Source: CAD feature listing. Evaluate the final solid. Frame: model axes, mm. Coordinates: 2 decimals unless noted, no trailing zeros. Order: outer loops, then holes, each group sorted by start corner. A loop starts at its lowest first (then second) coordinate and runs counter-clockwise, first axis right, second up. Notation, with made-up numbers: (64, -37) -> (78, -37) arc R12 ccw to (78, -23) -> close; hole circle Ø5 at (-24.5, 24.25). An arc over 180 degrees is marked (long way). Write item = value, one per line. Start each with the question number.
Item 1: Ray query, line 1 along Z through (x, y) = (-2.25, -0.25); line 2 along Y through (x, z) = (-2.5, 1.8); line 3 along Y through (x, z) = (0.5, 1.7). Return the intervals inside material, ascending. Write a range as [from, to].
Item 2: Section query B-B (y = 0). Output: boundary loops of the cut face in (x, z).
Item 3: Section query A-A (x = 0). Output: boundary loops of the cut face in (y, z), then the cut area to 3 significant figures.
```python
from build123d import *

# Parameters (mm, degrees)
SKETCH_R        = 15
PAD_DEPTH       = 1
PAD001_DEPTH    = 1
CHAMFER_SIZE    = 0.5
CHAMFER001_SIZE = 0.5


with BuildPart() as part:
    # Sketch → Pad (new body)
    with BuildSketch(Plane.XY):
        Circle(SKETCH_R)
    extrude(amount=PAD_DEPTH)

    # Sketch001 (on Face3 of Pad) → Pad001 (join)
    with BuildSketch(Plane.XY.offset(1)):
        Polygon((-12.321818, -1.832733), (-11.742344, -5.332733), (2.727027, -11.373328), (10.548595, 7.033819), (8.048595, 10.020412), (0.727027, -6.373328), align=None)
    extrude(amount=PAD001_DEPTH)

    # Chamfer
    chamfer_edges = [part.edges().sort_by_distance(p)[0] for p in [
        (-4.507658, -8.353031, 2),
        (-12.032081, -3.582733, 2),
        (-5.797395, -4.103031, 2),
        (4.387811, 1.823542, 2),
        (6.637811, -2.169755, 2),
        (9.298595, 8.527115, 2),
    ]]
    chamfer(chamfer_edges, length=CHAMFER_SIZE)

    # Chamfer001
    chamfer001_edges = [part.edges().sort_by_distance(p)[0] for p in [
        (-15, 0, 1),
    ]]
    chamfer(chamfer001_edges, length=CHAMFER001_SIZE)


solid = part.part
```
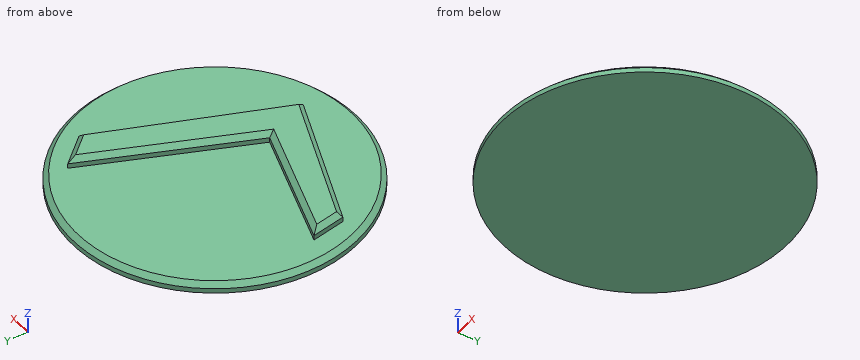
Computed:
q1.line_1 = [0, 1]
q1.line_2 = [-8.87, -5.57]
q1.line_3 = [-10.23, -6.51]
q2.outline = (-15, 0) -> (15, 0) -> (15, 0.5) -> (14.5, 1) -> (7.56, 1) -> (7.56, 1.5) -> (7.02, 2) -> (4.12, 2) -> (3.57, 1.5) -> (3.57, 1) -> (-14.5, 1) -> (-15, 0.5) -> close
q3.outline = (-15, 0) -> (15, 0) -> (15, 0.5) -> (14.5, 1) -> (-6.12, 1) -> (-6.12, 1.5) -> (-6.65, 2) -> (-9.69, 2) -> (-10.23, 1.5) -> (-10.23, 1) -> (-14.5, 1) -> (-15, 0.5) -> close
q3.area = 33.6 mm^2
